```python
from build123d import *

# Parameters (mm, degrees)
F0_R     = 11.303
F1_DEPTH = 7.239
F2_DEPTH = 25.4


with BuildPart() as f1:
    # F0 (on Top) → F1 (new body)
    with BuildSketch(Plane.XY):
        with BuildLine():
            ThreePointArc((-8.328858, 15.993502), (0, 12.83608), (8.328858, 15.993502))
            ThreePointArc((8.328858, 15.993502), (11.456334, 20.242046), (12.56392, 25.4))
            ThreePointArc((12.56392, 25.4), (-5.157954, 36.856334), (-8.328858, 15.993502))
        make_face()
        with Locations((0, 25.4)):
            Circle(F0_R, mode=Mode.SUBTRACT)
        with Locations((0, 25.4)):
            Circle(F0_R)
        with BuildLine():
            ThreePointArc((10.998523, 6.35), (12.267258, 3.287002), (12.7, 0))
            ThreePointArc((12.7, 0), (8.980256, -8.980256), (0, -12.7))
            Line((0, -12.7), (9.68635, -15.209754))
            ThreePointArc((9.68635, -15.209754), (11.116371, -6.41804), (18.015208, -0.783748))
            Line((18.015208, -0.783748), (10.998523, 6.35))
        make_face()
        with BuildLine():
            ThreePointArc((-10.998523, 6.35), (0, 12.7), (10.998523, 6.35))
            Line((10.998523, 6.35), (8.328858, 15.993502))
            ThreePointArc((8.328858, 15.993502), (0, 12.83608), (-8.328858, 15.993502))
            Line((-8.328858, 15.993502), (-10.998523, 6.35))
        make_face()
        with Locations((-21.997045, -12.7)):
            Circle(F0_R)
        with Locations((21.997045, -12.7)):
            Circle(F0_R)
        with BuildLine():
            ThreePointArc((0, -12.7), (8.980256, -8.980256), (12.7, 0))
            ThreePointArc((12.7, 0), (12.267258, 3.287002), (10.998523, 6.35))
            ThreePointArc((10.998523, 6.35), (0, 12.7), (-10.998523, 6.35))
            ThreePointArc((-10.998523, 6.35), (-10.998523, -6.35), (0, -12.7))
        make_face()
        Circle(F0_R, mode=Mode.SUBTRACT)
        Circle(F0_R)
        with BuildLine():
            ThreePointArc((34.560965, -12.7), (29.339545, -2.504914), (18.015208, -0.783748))
            ThreePointArc((18.015208, -0.783748), (11.116371, -6.41804), (9.68635, -15.209754))
            ThreePointArc((9.68635, -15.209754), (23.258293, -25.200453), (34.560965, -12.7))
        make_face()
        with Locations((21.997045, -12.7)):
            Circle(F0_R, mode=Mode.SUBTRACT)
        with BuildLine():
            ThreePointArc((-18.015208, -0.783748), (-32.877719, -18.98196), (-9.68635, -15.209754))
            ThreePointArc((-9.68635, -15.209754), (-9.496592, -13.961248), (-9.433125, -12.7))
            ThreePointArc((-9.433125, -12.7), (-11.801959, -5.3575), (-18.015208, -0.783748))
        make_face()
        with Locations((-21.997045, -12.7)):
            Circle(F0_R, mode=Mode.SUBTRACT)
        with BuildLine():
            Line((-9.68635, -15.209754), (0, -12.7))
            ThreePointArc((0, -12.7), (-10.998523, -6.35), (-10.998523, 6.35))
            Line((-10.998523, 6.35), (-18.015208, -0.783748))
            ThreePointArc((-18.015208, -0.783748), (-11.801959, -5.3575), (-9.433125, -12.7))
            ThreePointArc((-9.433125, -12.7), (-9.496592, -13.961248), (-9.68635, -15.209754))
        make_face()
    extrude(amount=F1_DEPTH)

    # F0 (on Top) → F2 (cut)
    with BuildSketch(Plane.XY):
        with Locations((21.997045, -12.7)):
            Circle(F0_R)
        Circle(F0_R)
        with Locations((0, 25.4)):
            Circle(F0_R)
        with Locations((-21.997045, -12.7)):
            Circle(F0_R)
    extrude(amount=F2_DEPTH, mode=Mode.SUBTRACT)


solid = f1.part
```
The listing builds one solid part. Answer for the finished solid, in the listing's coordinates (mm). A direction names the side the tool comes from. Give positions to 0.01 mm unless a question says otherwise; leave off trailing zeros. Loops run counter-clockwise (first coordinate to the right, second up) from the corner with the lowest first, then second, coordinate; pieces in that order, holes last. Notation, with made-up numbers: M 85.25,28.25 L 106.25,28.25 A31 cw 106.25,61.25 Z; hole C -30,76 d4. An arc over 180 degrees is marked long. One line per item, written item: value.
1. Section D-D on x = 7.5 is taken. Determine the outline of the cut face in (y, z), plus the area to 3 significant figures.
Found:
outline: M -14.64,0 L -8.46,0 L -8.46,7.24 L -14.64,7.24 Z; M 8.46,0 L 16.94,0 L 16.94,7.24 L 8.46,7.24 Z; M 33.86,0 L 35.48,0 L 35.48,7.24 L 33.86,7.24 Z
area: 118 mm^2
2. Each of these flat-tipped pins is pushed along its axis until it touches: P1, Ø3, axis at x = 16, z = 1.5, coming from the +Y side; P2, Ø1.5, axis at y = 13.5, z = 6, coming from the +X side. Where does it stop, or does it pass through?
Found:
P1: y = 2.79
P2: x = 9.23
3. Section B-B on z = 2.25 is taken. Determine the outline of the cut face in (x, y), plus the area to 3 significant figures.
Found:
outline: M -18.02,-0.78 A12.56 ccw long -9.69,-15.21 L 0,-12.7 L 9.69,-15.21 A12.56 ccw long 18.02,-0.78 L 11,6.35 L 8.33,15.99 A12.56 ccw 12.56,25.4 A12.56 ccw long -8.33,15.99 L -11,6.35 Z; hole C -22,-12.7 d22.61; hole C 0,0 d22.61; hole C 0,25.4 d22.61; hole C 22,-12.7 d22.61
area: 543 mm^2
4. For faces 1 (the face through (9.682, 11.104, 3.569)), 2 (the face through (-4.911, -13.972, 3.569)), 3 (the face through (-10.4, -5.2, 7.239)), determine the directions among +Z, -Z, +X, -X, +Y, -Y from which every point of the face is accessible in a straight line to the end or side of a thin tool.
Found:
face 1: +Z, -Z, +X
face 2: +Z, -Z, -Y
face 3: +Z, +X, -X, +Y, -Y
5. For a pull along Y with two mould halves and no side action, classify faces 4 (the face through (-9.645, 11.239, 3.569)), 5 (the face through (4.78, -13.94, 3.57)), 6 (the face through (-10.4, -5.2, 0)) as pulls with the +Y half, pulls with the -Y half, needs draft (parallel to the pull), parting line crosses it, or undercut.
Found:
face 4: undercut
face 5: pulls with the -Y half
face 6: needs draft
6. Find the intervals of material crossed by probe 1 along X at (y, z) = (25.4, 5.5); probe 2 along X at (y, z) = (26, 3.75); probe 3 along Y at (x, z) = (22.5, 1.5), in increasing order.
Found:
probe 1: -12.56 to -11.3, 11.3 to 12.56
probe 2: -12.55 to -11.29, 11.29 to 12.55
probe 3: -25.25 to -23.99, -1.41 to -0.15
7. Section A-A on y = -4.5 is taken. Determine the outline of the cut face in (x, z).
Found:
outline: M -31.52,0 L -29.78,0 L -29.78,7.24 L -31.52,7.24 Z; M -14.22,0 L -10.37,0 L -10.37,7.24 L -14.22,7.24 Z; M 10.37,0 L 14.22,0 L 14.22,7.24 L 10.37,7.24 Z; M 29.78,0 L 31.52,0 L 31.52,7.24 L 29.78,7.24 Z
8. Section C-C on x = 24.5 is taken. Determine the outline of the cut face in (y, z).
Found:
outline: M -25.01,0 L -23.72,0 L -23.72,7.24 L -25.01,7.24 Z; M -1.68,0 L -0.39,0 L -0.39,7.24 L -1.68,7.24 Z
